Design review of the part built by this model. Coordinates are the model's own, in mm. A direction names the side the tool comes from. Coordinates: 2 decimals unless noted, no trailing zeros. Loops run counter-clockwise (first coordinate to the right, second up) from the corner with the lowest first, then second, coordinate; pieces in that order, holes last. Notation, with made-up numbers: M -29,68.25 L 26,68.25 A19 ccw 26,72.25 Z; hole C 61,-25 d1. An arc over 180 degrees is marked long. One line per item, written item: value.
```python
from build123d import *

# Parameters (mm, degrees)
SKETCH_1_W          = 200
SKETCH_1_H          = 200
EXTRUDE_1_DEPTH     = 180
CHAMFER_1_SIZE      = 50
CHAMFER_1_SIZE2     = 86.602540378
SKETCH_2_R          = 27.5
EXTRUDE_2_DEPTH     = 20
EXTRUDE_START       = 20
SKETCH_2_3_R        = 32.5
SKETCH_2_3_R_2      = 27.5
EXTRUDE_3_DEPTH     = 8
FILLET_1_R          = 10
CUT_EXTRUDE_START   = -10
CUT_EXTRUDE_1_DEPTH = 180


with BuildPart() as part:
    # Sketch 1 → Extrude 1 (new body)
    with BuildSketch(Plane(origin=(0, 0, 0), x_dir=(1, 0, 0), z_dir=(0, 1, 0))):
        with Locations((100, 100)):
            Rectangle(SKETCH_1_W, SKETCH_1_H)
    extrude(amount=EXTRUDE_1_DEPTH)

    # Chamfer 1
    chamfer_1_edges = [part.edges().sort_by_distance(p)[0] for p in [
        (100, 180, 0),
    ]]
    chamfer_1_side = [part.faces().sort_by_distance(p)[0] for p in [
        (100, 90, 0),
    ]]
    chamfer(chamfer_1_edges, length=CHAMFER_1_SIZE, length2=CHAMFER_1_SIZE2, reference=chamfer_1_side[0])

    # Sketch 2 → Extrude 2 (add)
    with BuildSketch(Plane(origin=(0, 97.5, 56.291651246), x_dir=(1, 0, 0), z_dir=(0, 0.866025404, 0.5))):
        with Locations((100, 115)):
            Circle(SKETCH_2_R)
    extrude(amount=EXTRUDE_2_DEPTH)

    # Sketch 2_3 → Extrude 3 (add)
    with BuildSketch(Plane(origin=(0, 97.5, 56.291651246), x_dir=(1, 0, 0), z_dir=(0, 0.866025404, 0.5)).offset(EXTRUDE_START)):
        with Locations((100, 115)):
            Circle(SKETCH_2_3_R)
        with Locations((100, 115)):
            Circle(SKETCH_2_3_R_2, mode=Mode.SUBTRACT)
    extrude(amount=-EXTRUDE_3_DEPTH)

    # Fillet 1
    fillet_1_edges = [part.edges().sort_by_distance(p)[0] for p in [
        (100, 180, -200),
        (200, 180, -143.301270189),
        (100, 180, -86.602540378),
        (200, 65, 0),
        (200, 155, -43.301270189),
        (0, 65, 0),
        (100, 130, 0),
        (0, 155, -43.301270189),
        (72.5, 155, -43.301270189),
        (0, 180, -143.301270189),
        (100, 0, -200),
        (200, 0, -100),
        (100, 0, 0),
        (0, 0, -100),
        (0, 90, -200),
        (200, 90, -200),
    ]]
    fillet(fillet_1_edges, radius=FILLET_1_R)

    # Sketch 3 → Cut-Extrude 1 (cut)
    with BuildSketch(Plane(origin=(200, 0, 0), x_dir=(0, 0, -1), z_dir=(1, 0, 0)).offset(CUT_EXTRUDE_START)):
        Polygon((187, 13), (187, 167), (90.08587988, 167), (13, 122.494446501), (13, 13), align=None)
    extrude(amount=-CUT_EXTRUDE_1_DEPTH, mode=Mode.SUBTRACT)


solid = part.part
```
(1) We need section B-B on y = 106.5. State the section outline as (x, z) points.
Reply:
outline: M 0,-190 A10 ccw 10,-200 L 190,-200 A10 ccw 200,-190 L 200,-10 A10 ccw 190,0 L 10,0 A10 ccw 0,-10 Z; hole M 10,-187 L 190,-187 L 190,-13 L 10,-13 Z
(2) Tool access review of faces 1 (the flat face through (99, 180, -140)), 2 (the flat face through (190, 91, -99)), 3 (the flat face through (0, 89, -99)): name each direction out of +Z, -Z, +X, -X, +Y, -Y from which nothing blocks a thin tool from reaching the whole face with its end or side.
Reply:
face 1: -Z, +X, -X, +Y
face 2: none
face 3: +Z, -Z, -X, +Y, -Y
(3) To check wall thickness, follow line 1 along Z through (x, y) = (78, 74.5); line 2 along Y through (x, z) = (105.5, -92.5); line 3 along X through (y, z) = (78.5, -90). State the ranges of each line that lie inside material, in increasing order. Write a range as [from, to].
Reply:
line 1: z = [-200, -187], [-13, 0]
line 2: y = [0, 13], [167, 180]
line 3: x = [0, 10], [190, 200]
(4) Mouldability with a two-part tool opening along Y and no side actions: class faces 4 (the cylindrical face through (67.53, 169.62, -36.51)), 5 (the flat face through (99, 0, -101)), 6 (the cylindrical face through (197.15, 91.12, -196.99)) as released by +Y, released by -Y, zero draft, split by the parting line, or undercut.
Reply:
face 4: undercut
face 5: released by -Y
face 6: zero draft
(5) We need section A-A on z = -122.5. State the section outline as (x, y) points.
Reply:
outline: M 0,10 A10 ccw 10,0 L 190,0 A10 ccw 200,10 L 200,170 A10 ccw 190,180 L 10,180 A10 ccw 0,170 Z; hole M 10,13 L 190,13 L 190,167 L 10,167 Z
(6) We need section C-C on x = 143.5. State the section outline as (y, z) points.
Reply:
outline: M 0,-190 A10 ccw 10,-200 L 170,-200 A10 ccw 180,-190 L 180,-89.28 A10 ccw 178.66,-84.28 L 132.89,-5 A10 ccw 124.23,0 L 10,0 A10 ccw 0,-10 Z; hole M 13,-187 L 167,-187 L 167,-90.09 L 122.49,-13 L 13,-13 Z
(7) Insertion check: pin 1 (1 mm diameter, centred on x = 87, z = -85.5, fed in from +Y); pin 2 (4 mm diameter, centred on x = 29, z = -41, fed in from +Y); pin 3 (3 mm diameter, centred on x = 24.5, z = -174.5, fed in from +Y). Each pin has a flat end and moves straight along its axis. Give the tip position at first contact, or say it passes through.
Reply:
pin 1: stops at y = 179.45
pin 2: stops at y = 154.83
pin 3: stops at y = 180
